Geometry check sheet. Reference: the model listing, model coordinates, mm. Face numbers are marked on the shaded views. A direction names the side the tool comes from. Coordinates: 2 decimals unless noted, no trailing zeros. Order: outer loops, then holes, each group sorted by start corner. A loop starts at its lowest first (then second) coordinate and runs counter-clockwise, first axis right, second up. Notation, with made-up numbers: (22, 31.25) - (45, 31.25) arc R20 ccw to (45, 49.25) - close; hole circle Ø6 at (-27.75, 19.25). An arc over 180 degrees is marked (long way). Use CSV: the item, a comma, the result in double quotes. Start each with the question number.
1) Sectioned sample at A-A, the plane x = 22. Record the cut outline in (y, z), and give its area (3 significant figures).
2) Draft check along Z on the marked faces 3, 4 and 5. Enter one of: released by +Z, released by -Z, zero draft, split by the parting line, or undercut.
3) Depth check by flat-ended pin: P1, Ø1, axis at y = -21, z = 47, coming from the +X side; P2, Ø1.5, axis at x = 131.5, y = -15, coming from the +Z side; P3, Ø8, axis at x = -9.5, y = -11, coming from the +Z side; P4, Ø5, axis at x = 64, z = -16, coming from the +Y side. Enter the tip coordinate at first touch or a pass-through.
4) Thickness scan on probe 1 along X at (y, z) = (-11.5, 21.5); probe 2 along Z at (x, y) = (103, -11.25); probe 3 along Z at (x, y) = (107, -5.75). Record the ranges inside material, lowest first. Write a range as [from, to].
5) Tool access check on the marked faces 1 and 2. Record the directions out of +Z, -Z, +X, -X, +Y, -Y that give a thin tool (end or side, any length) a straight path to the whole face; none if there is none.
6) Sectioned sample at D-D, the plane z = -22. Record the cut outline in (x, y).
7) Sectioned sample at C-C, the plane z = 20.5. Record the cut outline in (x, y).
8) Sectioned sample at B-B, the plane y = -2.5. Record the cut outline in (x, z).
from build123d import *

# Parameters (mm, degrees)
F1_DEPTH = 25.4


with BuildPart() as f1:
    # F0 (on Front) → F1 (new body)
    with BuildSketch(Plane.XZ):
        Polygon((26.530553, 74.750386), (-53.061098, 6.366197), (13.146355, 6.366197), (36.734607, 24.124743), align=None)
        Polygon((13.146355, 6.366197), (-53.061098, 6.366197), (-53.061098, -43.478452), align=None)
        Polygon((122.448683, 6.366197), (13.146355, 6.366197), (-53.061098, -43.478452), (122.448683, -43.478452), align=None)
        Polygon((161.224097, 76.388255), (26.530553, 74.750386), (36.734607, 24.124743), (134.954938, 28.95045), align=None)
        Polygon((134.954938, 28.95045), (122.448683, 6.366197), (122.448683, -43.478452), (170.917973, 30.717365), align=None)
        Polygon((170.917973, 30.717365), (161.224097, 76.388255), (134.954938, 28.95045), align=None)
    extrude(amount=F1_DEPTH)


solid = f1.part
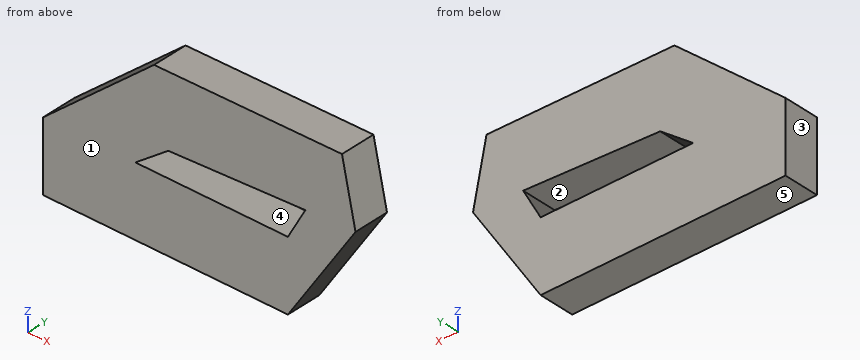
Evaluation:
1,outline,"(-25.4, -43.48) - (0, -43.48) - (0, 6.37) - (-25.4, 6.37) - close; (-25.4, 13.03) - (0, 13.03) - (0, 70.86) - (-25.4, 70.86) - close"
1,area,"2,730 mm²"
2,face 3,"zero draft"
2,face 4,"undercut"
2,face 5,"released by -Z"
3,P1,"x = 167.57"
3,P2,"z = 76.04"
3,P3,"z = 47.23"
3,P4,"y = 0"
4,probe 1,"[-35.45, 33.25], [130.83, 164.9]"
4,probe 2,"[-43.48, 6.37], [27.38, 75.68]"
4,probe 3,"[-43.48, 6.37], [27.58, 75.73]"
5,face 1,"+Z, -Z, +X, -X, -Y"
5,face 2,"+Y, -Y"
6,outline,"(-53.06, -25.4) - (136.48, -25.4) - (136.48, 0) - (-53.06, 0) - close"
7,outline,"(-36.61, -25.4) - (31.92, -25.4) - (31.92, 0) - (-36.61, 0) - close; (130.28, -25.4) - (164.24, -25.4) - (164.24, 0) - (130.28, 0) - close"
8,outline,"(-53.06, -43.48) - (122.45, -43.48) - (170.92, 30.72) - (161.22, 76.39) - (26.53, 74.75) - (-53.06, 6.37) - close; hole (13.15, 6.37) - (122.45, 6.37) - (134.95, 28.95) - (36.73, 24.12) - close"
